For this review, take the finished solid that the model builds, in its own axes (mm). A direction names the side the tool comes from. Coordinates: 2 decimals unless noted, no trailing zeros. Order: outer loops, then holes, each group sorted by start corner. A loop starts at its lowest first (then second) coordinate and runs counter-clockwise, first axis right, second up. Notation, with made-up numbers: M -17,24 L -6,24 A33 ccw -6,52 Z; hole C 9,-34 d5. An arc over 180 degrees is marked long. Use CSV: the item, a comma, the result in double quotes.
```python
from build123d import *

# Parameters (mm, degrees)
F1_DEPTH = 5
F3_DEPTH = 10
F4_DEPTH = 10


# Not quite as in the source:
# - a feature names something its author has since deleted; it is built from what else it names


with BuildPart() as f1:
    # F0 (on Top) → F1 (new body)
    with BuildSketch(Plane.XY):
        Polygon((290, -167.431578065), (0, 334.86315613), (-290, -167.431578065), align=None)
    extrude(amount=F1_DEPTH)

    # F2 (on face) → F3 (join)
    with BuildSketch(Plane.XY.offset(5)):
        with BuildLine():
            Line((256.3882985588, -141.2744761391), (-0.1700333609, 303.0975898508))
            Line((-0.1700333609, 303.0975898508), (-256.7283652805, -141.2744761391))
            Line((-256.7283652805, -141.2744761391), (-193.5489429105, -104.7978196266))
            Line((-193.5489429105, -104.7978196266), (-0.1700333609, 230.1442768257))
            Line((-0.1700333609, 230.1442768257), (193.2088761888, -104.7978196266))
            Line((193.2088761888, -104.7978196266), (-130.3695205406, -104.7978196266))
            Line((-130.3695205406, -104.7978196266), (-0.1700333609, 120.7143072881))
            Line((-0.1700333609, 120.7143072881), (98.6142485835, -50.3850880286))
            Line((98.6142485835, -50.3850880286), (18.3761417155, -50.3850880286))
            ThreePointArc((18.3761417155, -50.3850880286), (16.3865094235, -41.8600549069), (10.8287170908, -35.0964929185))
            Line((10.8287170908, -35.0964929185), (-12.5935137719, -35.0964929185))
            ThreePointArc((-12.5935137719, -35.0964929185), (-18.1513061046, -41.8600549069), (-20.1409383966, -50.3850880286))
            Line((-20.1409383966, -50.3850880286), (-20.1409383966, -86.5594913703))
            Line((-20.1409383966, -86.5594913703), (161.6191650039, -86.5594913703))
            Line((161.6191650039, -86.5594913703), (-0.1700333609, 193.6676203132))
            Line((-0.1700333609, 193.6676203132), (-193.5489429105, -141.2744761391))
            Line((-193.5489429105, -141.2744761391), (256.3882985588, -141.2744761391))
        make_face()
    extrude(amount=F3_DEPTH)

    # F2 (on face) → F4 (join)
    with BuildSketch(Plane.XY.offset(5)):
        with BuildLine():
            Line((-60.7889089023, -35.0964929185), (-12.5935137719, -35.0964929185))
            ThreePointArc((-12.5935137719, -35.0964929185), (-7.065251394, -32.1460175148), (-0.8823983405, -31.1265479726))
            ThreePointArc((-0.8823983405, -31.1265479726), (1.9162643927, -31.3309847436), (4.6555093745, -31.9399547076))
            ThreePointArc((4.6555093745, -31.9399547076), (1.2463845952, -2.8955610808), (27.1223774556, -16.5202418624))
            ThreePointArc((27.1223774556, -16.5202418624), (20.4987699273, -29.7504111213), (5.9377581342, -32.3746235496))
            ThreePointArc((5.9377581342, -32.3746235496), (8.4826511964, -33.5569208004), (10.8287170908, -35.0964929185))
            Line((10.8287170908, -35.0964929185), (60.7889089023, -35.0964929185))
            Line((60.7889089023, -35.0964929185), (0, 70.1929858369))
            Line((0, 70.1929858369), (-60.7889089023, -35.0964929185))
        make_face()
        with BuildLine():
            ThreePointArc((-0.8823983405, -31.1265479726), (-7.065251394, -32.1460175148), (-12.5935137719, -35.0964929185))
            Line((-12.5935137719, -35.0964929185), (10.8287170908, -35.0964929185))
            ThreePointArc((10.8287170908, -35.0964929185), (8.4826511964, -33.5569208004), (5.9377581342, -32.3746235496))
            ThreePointArc((5.9377581342, -32.3746235496), (5.2921802317, -32.1704267711), (4.6555093745, -31.9399547076))
            ThreePointArc((4.6555093745, -31.9399547076), (1.9162643927, -31.3309847436), (-0.8823983405, -31.1265479726))
        make_face()
    extrude(amount=F4_DEPTH)


solid = f1.part
```
Item 1: For faces 1 (the face through (-126.653, 84.022, 9.93)), 2 (the face through (48.53, 36.36, 9.93)), 3 (the face through (147.03, 80.2, 2.46)), list the 3-axis set-ups (+Z, -Z, +X, -X, +Y, -Y) from which the entire face can be reached by the end or side of a thin tool; tool diameter is ignored.
Solutions:
face 1,"+Z, -X, +Y"
face 2,"+Z"
face 3,"+Z, -Z, +X, +Y"
Item 2: Add section D-D on x = -38. State the section outline as (y, z) points, and give its area (3 significant figures).
Solutions:
outline,"M -167.43,0 L 269.05,0 L 269.05,5 L 237.57,5 L 237.57,15 L 164.62,15 L 164.62,5 L 128.14,5 L 128.14,15 L 55.19,15 L 55.19,5 L 4.38,5 L 4.38,15 L -35.1,15 L -35.1,5 L -104.8,5 L -104.8,15 L -141.27,15 L -141.27,5 L -167.43,5 Z"
area,"4,400 mm^2"
Item 3: Add section A-A on z = 10. State the section outline as (x, y) points.
Solutions:
outline,"M -256.73,-141.27 L -193.55,-104.8 L -0.17,230.14 L 193.21,-104.8 L -130.37,-104.8 L -0.17,120.71 L 98.61,-50.39 L 18.38,-50.39 A19.26 ccw 10.83,-35.1 L 60.79,-35.1 L 0,70.19 L -60.79,-35.1 L -12.59,-35.1 A19.26 ccw -20.14,-50.39 L -20.14,-86.56 L 161.62,-86.56 L -0.17,193.67 L -193.55,-141.27 L 256.39,-141.27 L -0.17,303.1 Z; hole C 10.6,-16.52 d33.05"
Item 4: Add section C-C on x = -209. State the section outline as (y, z) points, and give its area (3 significant figures).
Solutions:
outline,"M -167.43,0 L -27.14,0 L -27.14,5 L -58.61,5 L -58.61,15 L -113.72,15 L -113.72,5 L -167.43,5 Z"
area,"1,250 mm^2"
Item 5: To check wall thickness, follow line 1 along X through (y, z) = (125, 10); line 2 along X through (y, z) = (136, 12.5); line 3 along X through (y, z) = (-69, 8.5). State the ranges of each line that lie inside material, in increasing order. Write a range as [from, to].
Solutions:
line 1,"[-102.99, -60.88], [-39.82, 39.48], [60.54, 102.65]"
line 2,"[-96.64, -54.52], [-33.46, 33.12], [54.18, 96.3]"
line 3,"[-215, -172.88], [-151.82, -109.7], [-20.14, 151.48], [172.54, 214.66]"
Item 6: Add section B-B on y = -80. State the section outline as (x, z) points.
Solutions:
outline,"M -239.52,0 L 239.52,0 L 239.52,5 L 221.01,5 L 221.01,15 L 178.89,15 L 178.89,5 L 157.83,5 L 157.83,15 L -20.14,15 L -20.14,5 L -116.05,5 L -116.05,15 L -158.17,15 L -158.17,5 L -179.23,5 L -179.23,15 L -221.35,15 L -221.35,5 L -239.52,5 Z"
Item 7: Clearance check with flat-ended pins moving along their axes: pin 1 Ø4 at (y, z) = (113.5, 9) entering from +X; pin 2 Ø8 at (y, z) = (-69, 8) entering from -X; pin 3 Ø5 at (y, z) = (-45.5, 8.5) entering from +X. State where each tip first meets the part, or that it passes through.
Solutions:
pin 1,"x = 110.45"
pin 2,"x = -234.7"
pin 3,"x = 202.54"
Item 8: Draft analysis for pull direction Y (two halves, no side actions). For faces 4 (the face through (129.905, 77.801, 9.93)), 5 (the face through (10, -16, 5)), 6 (the face through (81.86, 51.59, 9.93)), 7 (the face through (-225.58, -123.29, 9.93)), state which applies: released by +Y, released by -Y, zero draft, split by the parting line, or undercut.
Solutions:
face 4,"released by +Y"
face 5,"undercut"
face 6,"undercut"
face 7,"released by -Y"
